Build history of the part. All positions in model axes, mm. Coordinates: 2 decimals unless noted, no trailing zeros. Order: outer loops, then holes, each group sorted by start corner. A loop starts at its lowest first (then second) coordinate and runs counter-clockwise, first axis right, second up. Notation, with made-up numbers: (-39.5, 67.25) - (-22.5, 67.25) arc R18 ccw to (-22.5, 89.25) - close; hole circle Ø8 at (49.25, -17). An arc over 180 degrees is marked (long way). One line per item, written item: value.
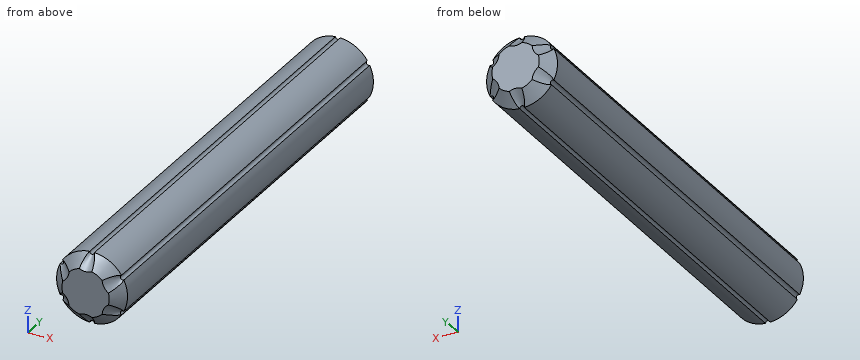
from build123d import *

# Parameters (mm, degrees)
SKETCH1_R           = 3
BOSS_EXTRUDE1_DEPTH = 40
CUT_EXTRUDE1_START  = -41
SKETCH2_R           = 0.2
CUT_EXTRUDE1_DEPTH  = 42
CIRPATTERN1_COUNT   = 6
CHAMFER1_SIZE       = 1


with BuildPart() as part:
    # Sketch1 → Boss-Extrude1 (new body)
    with BuildSketch(Plane(origin=(0, 0, 0), x_dir=(1, 0, 0), z_dir=(0, 1, 0))):
        Circle(SKETCH1_R)
    extrude(amount=BOSS_EXTRUDE1_DEPTH)

    # Sketch2 → Cut-Extrude1 (cut)
    with BuildSketch(Plane(origin=(0, 40, 0), x_dir=(1, 0, 0), z_dir=(0, 1, 0)).offset(CUT_EXTRUDE1_START)):
        with Locations((0, 3)):
            Circle(SKETCH2_R)
    cut_extrude1 = extrude(amount=CUT_EXTRUDE1_DEPTH, mode=Mode.SUBTRACT)

    # CirPattern1: Cut-Extrude1 ×6 about axis
    cirpattern1_axis = Axis((0, 0, 0), (0, 1, 0))
    for i in range(1, CIRPATTERN1_COUNT):
        add(cut_extrude1.rotate(cirpattern1_axis, i * 360 / CIRPATTERN1_COUNT), mode=Mode.SUBTRACT)

    # Chamfer1
    chamfer1_edges = [part.edges().sort_by_distance(p)[0] for p in [
        (-3, 0, 0),
        (-1.5, 0, 2.598076211),
        (1.5, 0, 2.598076211),
        (3, 0, 0),
        (1.5, 0, -2.598076211),
        (-2.424871131, 0, -1.4),
        (-2.424871131, 0, 1.4),
        (0, 0, 2.8),
        (2.424871131, 0, 1.4),
        (2.424871131, 0, -1.4),
        (-3, 40, 0),
        (-1.5, 40, 2.598076211),
        (1.5, 40, 2.598076211),
        (3, 40, 0),
        (1.5, 40, -2.598076211),
        (2.424871131, 40, -1.4),
        (2.424871131, 40, 1.4),
        (0, 40, 2.8),
        (-2.424871131, 40, 1.4),
        (-2.424871131, 40, -1.4),
        (-1.5, 0, -2.598076211),
        (0, 0, -2.8),
        (-1.5, 40, -2.598076211),
        (0, 40, -2.8),
    ]]
    chamfer(chamfer1_edges, length=CHAMFER1_SIZE)


solid = part.part
1. Probe line 1 along Z through (x, y) = (0.3, 14.5); line 2 along X through (y, z) = (14, 2.3); line 3 along Z through (x, y) = (2.6, 2). List the from-to ranges inside material, lowest first.
Values found:
line 1: z = -2.98 to 2.98
line 2: x = -1.93 to 1.93
line 3: z = -1.3 to 1.3
2. Band-saw the part on A-A, the plane y = 23. Give the cut face in (x, z), and give its area (3 significant figures).
Values found:
outline: (-2.69, -1.32) arc R0.2 cw to (-2.49, -1.67) arc R3 ccw to (-0.2, -2.99) arc R0.2 cw to (0.2, -2.99) arc R3 ccw to (2.49, -1.67) arc R0.2 cw to (2.69, -1.32) arc R3 ccw to (2.69, 1.32) arc R0.2 cw to (2.49, 1.67) arc R3 ccw to (0.2, 2.99) arc R0.2 cw to (-0.2, 2.99) arc R3 ccw to (-2.49, 1.67) arc R0.2 cw to (-2.69, 1.32) arc R3 ccw to start
area: 27.9 mm2
3. Flat gauge pins, fed straight in: P1, Ø1, axis at x = -1, y = 8, coming from the -Z side; P2, Ø3, axis at y = 25.5, z = 2, coming from the +X side. Where does each tip first touch, or does it go through?
Values found:
P1: stops at z = -2.96
P2: stops at x = 2.96
